The drawing under review shows one solid part. Ordinate dimensions are in mm from its lowest x, y, z. Give positions to 0.01 mm unless a question says otherwise; leave off trailing zeros. Order: outer loops, then holes, each group sorted by start corner. A loop starts at its lowest first (then second) coordinate and runs counter-clockwise, first axis right, second up. Notation, with made-up numbers: (-29.5, 69) -> (-3.5, 69) arc R24 ccw to (-3.5, 84) -> close; hole circle Ø1 at (-23.75, 5.25). An arc over 180 degrees is marked (long way). One line per item, written item: value. Start each with the question number.
1) Consider section B-B (z = 45). State the section outline as (x, y) points, plus the area to 3 significant figures.
2) Wall thickness on line 1 along X through (y, z) = (3.5, 15); line 2 along X through (y, z) = (3, 13.5): over which ranges is each line inside the solid? List them lowest first. Write a range as from..to.
3) For pin 1 (8 mm diameter, centred on x = 45, z = 15, fed in from -Y), flat-tipped, find the tip position at first contact; note if it passes through.
4) Consider section A-A (x = 15). State the section outline as (y, z) points, plus the area to 3 significant figures.
5) Consider section C-C (y = 8.5). State the section outline as (x, z) points.
6) The part is to be moulded in two halves that separate along Z. For the marked faces 1, 2, 3 and 4, say which applies: released by +Z, released by -Z, zero draft, split by the parting line, or undercut.
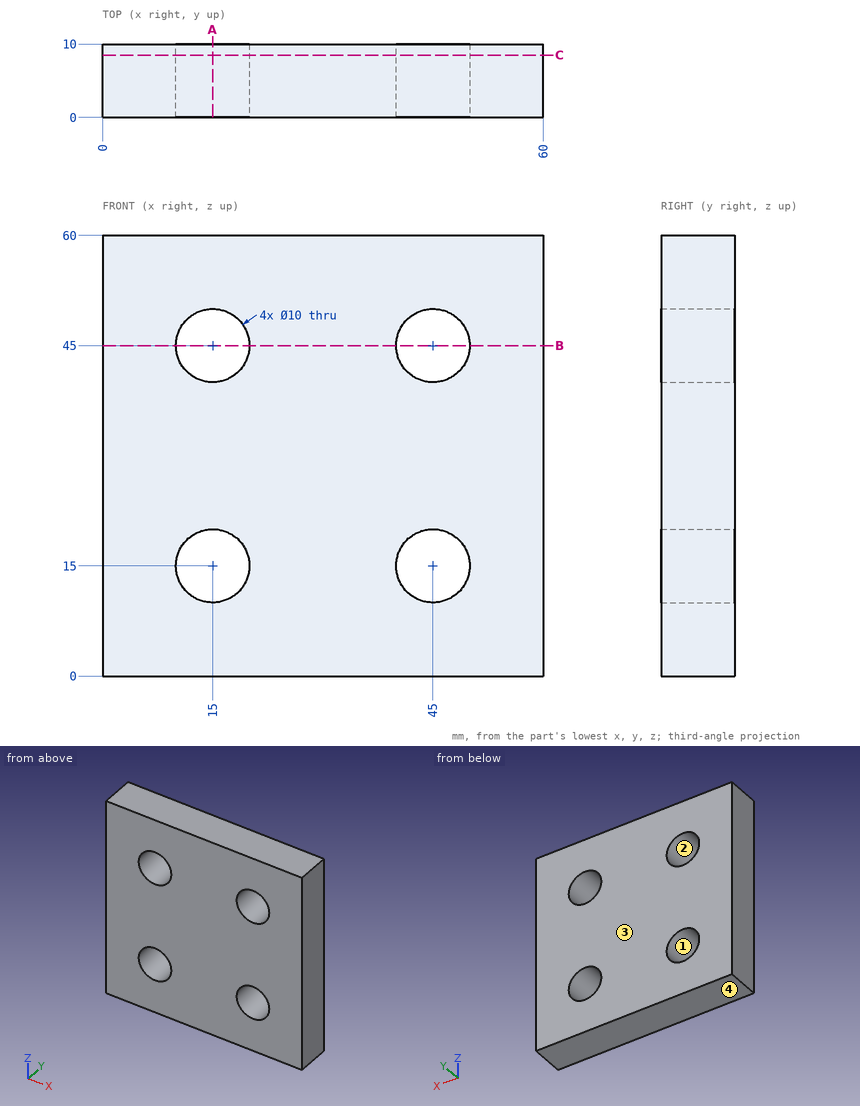
Checked values:
1. outline: (0, 0) -> (10, 0) -> (10, 10) -> (0, 10) -> close; (20, 0) -> (40, 0) -> (40, 10) -> (20, 10) -> close; (50, 0) -> (60, 0) -> (60, 10) -> (50, 10) -> close
1. area: 400 mm^2
2. line 1: x = 0..10, 20..40, 50..60
2. line 2: x = 0..10.23, 19.77..40.23, 49.77..60
3. pin 1: passes through
4. outline: (0, 0) -> (10, 0) -> (10, 10) -> (0, 10) -> close; (0, 20) -> (10, 20) -> (10, 40) -> (0, 40) -> close; (0, 50) -> (10, 50) -> (10, 60) -> (0, 60) -> close
4. area: 400 mm^2
5. outline: (0, 0) -> (60, 0) -> (60, 60) -> (0, 60) -> close; hole circle Ø10 at (15, 15); hole circle Ø10 at (15, 45); hole circle Ø10 at (45, 15); hole circle Ø10 at (45, 45)
6. face 1: undercut
6. face 2: undercut
6. face 3: zero draft
6. face 4: released by -Z
